from build123d import *

# Parameters (mm, degrees)
SKETCH_1_W                = 50.28
SKETCH_1_H                = 34.2
SKETCH_1_W_2              = 30.28
SKETCH_1_H_2              = 14.2
EXTRUDE_1_DEPTH           = 12.25
SKETCH_4_W                = 13
SKETCH_4_H                = 13.91
EXTRUDE_1_2_DEPTH         = 74.82
SKETCH_5_W                = 13.91
SKETCH_5_H                = 16.23
EXTRUDE_2_DEPTH           = 16
SKETCH_7_R                = 25.25
SKETCH_7_R_2              = 15.25
EXTRUDE_2_2_DEPTH         = 16.23
SKETCH_15_R               = 1.91
CUT_EXTRUDE_6_DEPTH       = 97.964478439
SKETCH_18_W               = 49.344544624
SKETCH_18_H               = 6.125
CUT_EXTRUDE_8_DEPTH       = 101.789238284
SKETCH_19_W               = 34.2
SKETCH_19_H               = 6.125
CUT_EXTRUDE_9_DEPTH       = 10
SKETCH_21_R               = 1.91
CUT_EXTRUDE_10_DEPTH      = 10
SKETCH_20_R               = 1.91
CUT_EXTRUDE_11_DEPTH      = 10
FILLET_START              = -7.1
FILLET_1_DEPTH            = 14.2
FILLET_2_DEPTH            = 14.2
SKETCH_29_W               = 13.91
SKETCH_29_H               = 74.82
EXTRUDE_5_DEPTH           = 10
SKETCH_30_W               = 10
SKETCH_30_H               = 58.59
CUT_EXTRUDE_13_DEPTH      = 97.964478439
SKETCH_32_W               = 34.2
SKETCH_32_H               = 5.745736365
EXTRUDE_6_DEPTH           = 10
CUT_EXTRUDE_16_DEPTH      = 50
CUT_EXTRUDE_16_DEPTH_BACK = 50
SKETCH_38_W               = 116.985630298
SKETCH_38_H               = 80.538350638
SKETCH_41_W               = 13.91
SKETCH_41_H               = 5.745736365
EXTRUDE_7_DEPTH           = 3
SKETCH_42_W               = 13
SKETCH_42_H               = 13.91
EXTRUDE_8_DEPTH           = 74.82
SKETCH_43_W               = 13.91
SKETCH_43_H               = 16.23
EXTRUDE_9_DEPTH           = 15.22
SKETCH_44_R               = 1.91
CUT_EXTRUDE_17_DEPTH      = 15.22
SKETCH_46_R               = 25.25
SKETCH_46_R_2             = 15.25
EXTRUDE_6_2_DEPTH         = 16.23
EXTRUDE_10_DEPTH          = 7.22
EXTRUDE_10_DEPTH_BACK     = 10
SKETCH_47_W               = 13.91
SKETCH_47_H               = 16.23
SKETCH_50_W               = 3.056753925
SKETCH_50_H               = 16.23
CUT_EXTRUDE_18_DEPTH      = 96.578211037
SKETCH_51_R               = 1.91
CUT_EXTRUDE_19_DEPTH      = 95.015226304
SKETCH_52_W               = 92.841945613
SKETCH_52_H               = 30
CUT_EXTRUDE_20_DEPTH      = 84.840694713


with BuildPart() as part:
    # 草圖1 → Extrude 1 (new body)
    with BuildSketch(Plane(origin=(0, 0, 0), x_dir=(1, 0, 0), z_dir=(0, 1, 0))):
        Rectangle(SKETCH_1_W, SKETCH_1_H)
        Rectangle(SKETCH_1_W_2, SKETCH_1_H_2, mode=Mode.SUBTRACT)
    extrude(amount=EXTRUDE_1_DEPTH)

    # 草圖4 → Extrude 1 2 (add)
    with BuildSketch(Plane.XZ):
        with Locations((18.64, 0)):
            Rectangle(SKETCH_4_W, SKETCH_4_H)
    extrude(amount=EXTRUDE_1_2_DEPTH)

    # 草圖5 → Extrude 2 (add)
    with BuildSketch(Plane.ZY.offset(-12.14)):
        with Locations((0, -66.705)):
            Rectangle(SKETCH_5_W, SKETCH_5_H)
    extrude(amount=EXTRUDE_2_DEPTH)

    # 草圖7 → Extrude 2 2 (add)
    with BuildSketch(Plane(origin=(3.626674765, -74.82, 0), x_dir=(1, 0, 0), z_dir=(0, -1, 0))):
        with Locations((-30.978154344, 0)):
            Circle(SKETCH_7_R)
        with Locations((-30.978154344, 0)):
            Circle(SKETCH_7_R_2, mode=Mode.SUBTRACT)
    extrude(amount=-EXTRUDE_2_2_DEPTH)

    # 草圖15 → 除料-伸長6 (cut, through all)
    with BuildSketch(Plane(origin=(0, 0, -6.955), x_dir=(-1, 0, 0), z_dir=(0, 0, -1))):
        with Locations((-4.530883248, -66.705)):
            Circle(SKETCH_15_R)
    extrude(amount=-CUT_EXTRUDE_6_DEPTH, mode=Mode.SUBTRACT)

    # 草圖18 → 除料-伸長8 (cut, through all)
    with BuildSketch(Plane(origin=(0, 0, -17.1), x_dir=(-1, 0, 0), z_dir=(0, 0, -1))):
        with Locations((0.467727688, 9.1875)):
            Rectangle(SKETCH_18_W, SKETCH_18_H)
    extrude(amount=-CUT_EXTRUDE_8_DEPTH, mode=Mode.SUBTRACT)

    # 草圖19 → 除料-伸長9 (cut)
    with BuildSketch(Plane.ZY.offset(-24.204544624)):
        with Locations((0, 9.1875)):
            Rectangle(SKETCH_19_W, SKETCH_19_H)
    extrude(amount=-CUT_EXTRUDE_9_DEPTH, mode=Mode.SUBTRACT)

    # 草圖21 → 除料-伸長10 (cut)
    with BuildSketch(Plane(origin=(0, 6.125, 0), x_dir=(1, 0, 0), z_dir=(0, 1, 0))):
        with Locations(Location((17.69, 0, 0), (0, 0, 270))):
            Circle(SKETCH_21_R)
    extrude(amount=-CUT_EXTRUDE_10_DEPTH, mode=Mode.SUBTRACT)

    # 草圖20 → 除料-伸長11 (cut)
    with BuildSketch(Plane(origin=(0, 6.125, 0), x_dir=(1, 0, 0), z_dir=(0, 1, 0))):
        with Locations(Location((-17.395, 0, 0), (0, 0, 270))):
            Circle(SKETCH_20_R)
    extrude(amount=-CUT_EXTRUDE_11_DEPTH, mode=Mode.SUBTRACT)

    # 圓角1: read off the stored shape, not the designer's step
    # 圓角1 outline → 圓角1 (cut)
    with BuildSketch(Plane.XY.offset(FILLET_START)):
        with BuildLine():
            add(Edge.make_bspline(
                [(-15.14, 0), (-21.974170252, 5.199829476), (-25.14, 5.745736365)],
                knots=[0, 0, 0, 0.664102345, 0.664102345, 0.664102345], degree=2, weights=[1, 2.223777218, 1.822127795]))
            Line((-15.14, 0), (-15.14, 6.125))
            Line((-15.14, 6.125), (-25.14, 6.125))
            Line((-25.14, 6.125), (-25.14, 5.745736365))
        make_face()
    extrude(amount=FILLET_1_DEPTH, mode=Mode.SUBTRACT)

    # 圓角2: read off the stored shape, not the designer's step
    # 圓角2 outline → 圓角2 (cut)
    with BuildSketch(Plane.XY.offset(FILLET_START)):
        with BuildLine():
            Line((15.14, 6.125), (15.14, 0))
            add(Edge.make_bspline(
                [(15.14, 0), (21.974170252, 5.199829476), (25.14, 5.745736365)],
                knots=[0, 0, 0, 0.664102345, 0.664102345, 0.664102345], degree=2, weights=[1, 2.223777218, 1.822127795]))
            Line((25.14, 5.745736365), (25.14, 6.125))
            Line((25.14, 6.125), (15.14, 6.125))
        make_face()
    extrude(amount=FILLET_2_DEPTH, mode=Mode.SUBTRACT)

    # 草圖29 → 填料-伸長5 (add)
    with BuildSketch(Plane(origin=(25.14, 0, 0), x_dir=(0, 0, -1), z_dir=(1, 0, 0))):
        with Locations((0, -37.41)):
            Rectangle(SKETCH_29_W, SKETCH_29_H)
    extrude(amount=EXTRUDE_5_DEPTH)

    # 草圖30 → 除料-伸長13 (cut, through all)
    with BuildSketch(Plane.XY.offset(6.955)):
        with Locations((17.14, -29.295)):
            Rectangle(SKETCH_30_W, SKETCH_30_H)
    extrude(amount=-CUT_EXTRUDE_13_DEPTH, mode=Mode.SUBTRACT)

    # 草圖32 → Extrude 6 (add)
    with BuildSketch(Plane(origin=(25.14, 0, 0), x_dir=(0, 0, -1), z_dir=(1, 0, 0))):
        with Locations((0, 2.872868182)):
            Rectangle(SKETCH_32_W, SKETCH_32_H)
    extrude(amount=EXTRUDE_6_DEPTH)

    # 草圖38 → 除料-伸長16 (cut, two sides: drawn at the far end of the back side and taken through both)
    with BuildSketch(Plane(origin=(0, 0, -6.955), x_dir=(-1, 0, 0), z_dir=(0, 0, -1)).offset(-CUT_EXTRUDE_16_DEPTH_BACK)):
        with Locations((7.268869252, -40.269175319)):
            Rectangle(SKETCH_38_W, SKETCH_38_H)
    extrude(amount=CUT_EXTRUDE_16_DEPTH + CUT_EXTRUDE_16_DEPTH_BACK, mode=Mode.SUBTRACT)

    # 草圖41 → 填料-伸長7 (add)
    with BuildSketch(Plane(origin=(35.14, 0, 0), x_dir=(0, 0, -1), z_dir=(1, 0, 0))):
        with Locations((0, 2.872868182)):
            Rectangle(SKETCH_41_W, SKETCH_41_H)
    extrude(amount=EXTRUDE_7_DEPTH)

    # 草圖42 → 填料-伸長8 (add)
    with BuildSketch(Plane(origin=(0, 0, 0), x_dir=(-1, 0, 0), z_dir=(0, -1, 0))):
        with Locations((-31.64, 0)):
            Rectangle(SKETCH_42_W, SKETCH_42_H)
    extrude(amount=EXTRUDE_8_DEPTH)

    # 草圖43 → 填料-伸長9 (add)
    with BuildSketch(Plane.ZY.offset(-25.14)):
        with Locations((0, -66.705)):
            Rectangle(SKETCH_43_W, SKETCH_43_H)
    extrude(amount=EXTRUDE_9_DEPTH)

    # 草圖44 → 除料-伸長17 (cut)
    with BuildSketch(Plane(origin=(0, 0, -6.955), x_dir=(-1, 0, 0), z_dir=(0, 0, -1))):
        with Locations(Location((-17.524895264, -66.705, 0), (0, 0, 90))):
            Circle(SKETCH_44_R)
    extrude(amount=-CUT_EXTRUDE_17_DEPTH, mode=Mode.SUBTRACT)

    # 草圖46 → Extrude 6 2 (add)
    with BuildSketch(Plane(origin=(0, -58.59, 0), x_dir=(1, 0, 0), z_dir=(0, 1, 0))):
        with Locations((-14.35, 0)):
            Circle(SKETCH_46_R)
        with Locations((-14.35, 0)):
            Circle(SKETCH_46_R_2, mode=Mode.SUBTRACT)
    extrude(amount=-EXTRUDE_6_2_DEPTH)

    # 草圖47 → 填料-伸長10 (add, two sides: drawn at the far end of the back side and taken through both)
    with BuildSketch(Plane(origin=(-40, 0, 0), x_dir=(0, 0, -1), z_dir=(1, 0, 0)).offset(-EXTRUDE_10_DEPTH_BACK)):
        with Locations((0, -66.705)):
            Rectangle(SKETCH_47_W, SKETCH_47_H)
    extrude(amount=EXTRUDE_10_DEPTH + EXTRUDE_10_DEPTH_BACK)

    # 草圖50 → 除料-伸長18 (cut, through all)
    with BuildSketch(Plane(origin=(0, 0, -6.955), x_dir=(-1, 0, 0), z_dir=(0, 0, -1))):
        with Locations((48.471623038, -66.705)):
            Rectangle(SKETCH_50_W, SKETCH_50_H)
    extrude(amount=-CUT_EXTRUDE_18_DEPTH, mode=Mode.SUBTRACT)

    # 草圖51 → 除料-伸長19 (cut, through all)
    with BuildSketch(Plane(origin=(0, 0, -6.955), x_dir=(-1, 0, 0), z_dir=(0, 0, -1))):
        with Locations((42.786508152, -66.705)):
            Circle(SKETCH_51_R)
    extrude(amount=-CUT_EXTRUDE_19_DEPTH, mode=Mode.SUBTRACT)

    # 草圖52 → 除料-伸長20 (cut, through all)
    with BuildSketch(Plane(origin=(0, -58.59, 0), x_dir=(1, 0, 0), z_dir=(0, 1, 0))):
        with Locations((-21.280972807, 15)):
            Rectangle(SKETCH_52_W, SKETCH_52_H)
    extrude(amount=-CUT_EXTRUDE_20_DEPTH, mode=Mode.SUBTRACT)


solid = part.part
CAD build for the part. Positions are in the model's coordinates, mm. A direction names the side the tool comes from. Coordinates: 2 decimals unless noted, no trailing zeros. Write each loop counter-clockwise with the first axis right and the second up, starting at its lowest first coordinate (ties: lowest second). Pieces come first, ordered by that corner, then holes. Notation, with made-up numbers: M 30.5,-23 L 68.5,-23 A32 cw 68.5,9 Z; hole C 71.25,-8.5 d8. An arc over 180 degrees is marked long. Answer as a JSON object with one key per item and string values. Group by question number.
1) Tool access for faces 5 (the face through (30, 5.746, 0)), 6 (the face through (35.14, 3, -12)), 7 (the face through (-11, -58.59, 16)): list every direction of +Z, -Z, +X, -X, +Y, -Y with a clear straight run to the whole face (end or side of a thin tool).
2) Wall check: line 1 (Z direction, x = 17.69, y = 2.2); line 2 (Y direction, x = -24, z = 13) (3 decimals); line 3 (Z direction, x = 32.5, y = -21) (3 decimals). Give the ranges that are in metal, low to high. Write a range as from..to.
3) Pin check, flat tips, straight feed: pin 1 Ø4 at (x, y) = (-41.5, -65) entering from +Z (3 decimals); pin 2 Ø3.5 at (x, z) = (17.69, 0) entering from +Y; pin 3 Ø3.5 at (x, y) = (17.52, -66.7) entering from -Z; pin 4 Ø8 at (x, y) = (-40.5, -67) entering from -Z. Stop position of each tip, or through.
4) Saw through at A-A (x = 30). Write the cut outline in (y, z) (3 decimals).
5) Saw through at C-C (x = -14). Write the cut outline in (y, z) (3 decimals), plus the area to 3 significant figures.
6) Saw through at B-B (y = -70). Write the cut outline in (x, z) (3 decimals), plus the area to 3 significant figures.
7) Saw through at D-D (x = -2). Write the cut outline in (y, z) (1 decimal), plus the area to 3 significant figures.
8) Mould opens along Y. For faces 1 (the face through (-1, -74.82, 12)), 2 (the face through (0, 6.125, 12)), 3 (the face through (17.609, -68.613, 3.429)), 4 (the face through (-25.14, 3, 0)) say: +Y half, -Y half, draft (parallel to the pull), parting line (faces both ways), or undercut.
Values follow:
{
 "1": {"face 5": "+Z, -Z, +X, +Y", "face 6": "-Z, +X, +Y, -Y", "face 7": "+Z, -Z, -X"},
 "2": {"line 1": "z = -17.1..-7.1, 7.1..17.1", "line 2": "y = -74.82..-58.59, 0..6.125", "line 3": "z = -6.955..6.955"},
 "3": {"pin 1": "stops at z = 6.955", "pin 2": "stops at y = -58.59", "pin 3": "passes through", "pin 4": "stops at z = 0"},
 "4": {"outline": "M -74.82,-6.955 L 0,-6.955 L 0,-17.1 L 5.746,-17.1 L 5.746,17.1 L 0,17.1 L 0,6.955 L -74.82,6.955 Z"},
 "5": {"outline": "M -74.82,15.246 L -58.59,15.246 L -58.59,25.248 L -74.82,25.248 Z; M 0,-17.1 L 6.125,-17.1 L 6.125,-7.1 L 0,-7.1 Z; M 0,7.1 L 6.125,7.1 L 6.125,17.1 L 0,17.1 Z", "area": "285 mm2"},
 "6": {"outline": "M -46.943,0 L -29.6,0 A15.25 cw 0.9,0 L 25.14,0 L 25.14,-6.955 L 38.14,-6.955 L 38.14,6.955 L 9.923,6.955 A25.25 ccw -38.623,6.955 L -46.943,6.955 Z", "area": "972 mm2"},
 "7": {"outline": "M -74.8,8.9 L -58.6,8.9 L -58.6,22 L -74.8,22 Z; M 0,-17.1 L 6.1,-17.1 L 6.1,-7.1 L 0,-7.1 Z; M 0,7.1 L 6.1,7.1 L 6.1,17.1 L 0,17.1 Z", "area": "335 mm2"},
 "8": {"face 1": "-Y half", "face 2": "+Y half", "face 3": "undercut", "face 4": "draft"}
}
